Autodesk Inventor part; units mm, degrees
ref_plane "YZ Plane" through (0, 0, 0) normal (1, 0, 0) x (0, 1, 0)
ref_plane "XZ Plane" through (0, 0, 0) normal (0, 1, 0) x (-1, 0, 0)
ref_plane "XY Plane" through (0, 0, 0) normal (0, 0, 1) x (1, 0, 0)
sketch "Esquisse1" plane through (0, 0, 0) normal (0, 1, 0) x (-1, 0, 0)
  line L0 (0, -4.0415) -> (-3.5, -2.0207)
  line L1 (-3.5, -2.0207) -> (-3.5, 2.0207)
  line L2 (-3.5, 2.0207) -> (0, 4.0415)
  line L3 (0, 4.0415) -> (3.5, 2.0207)
  line L4 (3.5, 2.0207) -> (3.5, -2.0207)
  line L5 (3.5, -2.0207) -> (0, -4.0415)
  point P0 (0, 0)
  point P1 (0, 0)
  dimension "d0" = 7
extrude "Extrusion1" add sketch "Esquisse1" along normal blind 50
sketch "Esquisse2" plane through (0, 0, 0) normal (0, -1, 0) x (1, 0, 0)
  circle A0 centre (0, 0) radius 2
  dimension "d3" = 4
extrude "Extrusion2" cut sketch "Esquisse2" against normal blind 10
sketch "Esquisse3" plane through (0, 50, 0) normal (0, 1, 0) x (1, 0, 0)
  circle A0 centre (0, 0) radius 2
  dimension "d6" = 4
extrude "Extrusion3" cut sketch "Esquisse3" against normal blind 10
thread "Filetage1"
thread "Filetage2"
properties part number "Entretoise-50mm" material "Acier"
Could you check a few things on this model? Use its own coordinates, in mm. A direction names the side the tool comes from. Give positions to 0.01 mm unless a question says otherwise; leave off trailing zeros. Order: outer loops, then holes, each group sorted by start corner. A loop starts at its lowest first (then second) coordinate and runs counter-clockwise, first axis right, second up. Notation, with made-up numbers: (-22.5, 23.5) - (18.5, 23.5) arc R20 cw to (18.5, 33.5) - close; hole circle Ø5 at (84, -17). An arc over 180 degrees is marked (long way). One line per item, written item: value. Start each with the question number.
1. Imagine slicing it at B-B on z = 0. List the corners of the cut face in (x, y) for me.
2. If I drill on probe 1 along Z at (x, y) = (0, 47.5); probe 2 along X at (y, z) = (44.5, 0); probe 3 along X at (y, z) = (8, 1), over which ranges is the centre line in solid material (lowest first)?
3. Thinking about a two-plate mould opening in X: for faces 4 (the face through (0, 5, -2)), 5 (the face through (1.8, 24.6, 3)), 6 (the face through (-1.8, 24.6, -3)), which applies, +X half, -X half, draft (parallel to the pull), parting line (faces both ways), or undercut?
4. For faces 1 (the face through (0, 45, 2)), 2 (the face through (0, 10, 0)), 3 (the face through (-1.726, 24.65, 3.045)), which set-ups out of +Z, -Z, +X, -X, +Y, -Y let a thin tool reach every point of the face, with its end or its side?
5. Imagine slicing it at C-C on x = 0.5. List the corners of the cut face in (y, z) for me.
6. Imagine slicing it at D-D on y = 20.5. List the corners of the cut face in (x, z) for me.
7. Imagine slicing it at A-A on y = 45.5. List the corners of the cut face in (x, z) for me.
8. For P1, Ø1.2, axis at x = -0.5, z = 1, coming from the -Y side, with a flat end and sliding along its axis, tell me the tip position at first contact or that it passes through.
Values:
1. outline: (-3.5, 0) - (-2, 0) - (-2, 10) - (2, 10) - (2, 0) - (3.5, 0) - (3.5, 50) - (2, 50) - (2, 40) - (-2, 40) - (-2, 50) - (-3.5, 50) - close
2. probe 1: -4.04 to -2, 2 to 4.04
2. probe 2: -3.5 to -2, 2 to 3.5
2. probe 3: -3.5 to -1.73, 1.73 to 3.5
3. face 4: undercut
3. face 5: +X half
3. face 6: -X half
4. face 1: +Y
4. face 2: -Y
4. face 3: +Z, -X, +Y, -Y
5. outline: (0, -3.75) - (50, -3.75) - (50, -1.94) - (40, -1.94) - (40, 1.94) - (50, 1.94) - (50, 3.75) - (0, 3.75) - (0, 1.94) - (10, 1.94) - (10, -1.94) - (0, -1.94) - close
6. outline: (-3.5, -2.02) - (0, -4.04) - (3.5, -2.02) - (3.5, 2.02) - (0, 4.04) - (-3.5, 2.02) - close
7. outline: (-3.5, -2.02) - (0, -4.04) - (3.5, -2.02) - (3.5, 2.02) - (0, 4.04) - (-3.5, 2.02) - close; hole circle Ø4 at (0, 0)
8. P1: y = 10
